Build history of the part. All positions in model axes, mm. A direction names the side the tool comes from. Give positions to 0.01 mm unless a question says otherwise; leave off trailing zeros. Write each loop counter-clockwise with the first axis right and the second up, starting at its lowest first coordinate (ties: lowest second). Pieces come first, ordered by that corner, then holes. Notation, with made-up numbers: (78, 89.5) -> (86, 89.5) arc R37 ccw to (86, 126.5) -> close; hole circle Ø8 at (17, 73). An arc over 180 degrees is marked (long way). One line per question, with ' | ' between items. Start each with the question number.
(1) Band-saw the part on B-B, the plane z = 0. Give the cut face in (x, y), and give its area (3 significant figures).
(2) Band-saw the part on C-C, the plane y = 5.5. Give the cut face in (x, z), and give its area (3 significant figures).
(3) Tool access for faces 4 (the cylindrical face through (0.03, 3.44, 7.66)), 5 (the flat face through (8, 14, -1.102)), 6 (the cylindrical face through (-5.323, 13.804, 2.769)): list every direction of +Z, -Z, +X, -X, +Y, -Y with a clear straight run to the whole face (end or side of a thin tool).
(4) Pull direction X, two halves, no side cores. Call faces 1 (the cylindrical face through (-0.027, 23.206, -7.713)), 2 (the cylindrical face through (-7.72, 3.79, -0.02)), 3 (the cylindrical face through (-3.639, 13.819, 8.776)): released by +X, released by -X, zero draft, split by the parting line, or undercut.
(5) Pin check, flat tips, straight feed: P1, Ø5, axis at x = 2.5, y = 7.5, coming from the -Z side; P2, Ø1.8, axis at x = -8.5, y = 15.5, coming from the -Z side; P3, Ø8, axis at y = 13, z = 5.5, coming from the -X side; P4, Ø2, axis at x = 4.5, z = 1, coming from the +Y side. Stop position of each tip, or through.
(6) Drill centre lines: probe 1 along X at (y, z) = (15.5, -7.5); probe 2 along Z at (x, y) = (-7.5, 11.25); probe 3 along Z at (x, y) = (2.25, 25.25). Where is each one in solid material? Low to high. Write a range as from..to.
(7) Band-saw the part on A-A, the plane x = 0. Give the cut face in (y, z), and give its area (3 significant figures).
from build123d import *

# Parameters (mm, degrees)
SKETCH_1_R               = 9.5
SKETCH_1_R_2             = 6
EXTRUDE_1_DEPTH          = 28
FILLET_1_R               = 1.1
CUT_EXTRUDE_1_DEPTH      = 15
CUT_EXTRUDE_1_DEPTH_BACK = 17
CUT_EXTRUDE_2_DEPTH      = 17
CUT_EXTRUDE_2_DEPTH_BACK = 17


with BuildPart() as part:
    # Эскиз1 → Бобышка-Вытянуть1 (new body)
    with BuildSketch(Plane(origin=(0, 0, 0), x_dir=(1, 0, 0), z_dir=(0, 1, 0))):
        with Locations(Location((0, 0, 0), (0, 0, 270))):
            Circle(SKETCH_1_R)
        with Locations(Location((0, 0, 0), (0, 0, 270))):
            Circle(SKETCH_1_R_2, mode=Mode.SUBTRACT)
    extrude(amount=EXTRUDE_1_DEPTH)

    # Скругление1
    fillet_1_edges = [part.edges().sort_by_distance(p)[0] for p in [
        (0, 0, -9.5),
        (0, 28, -9.5),
    ]]
    fillet(fillet_1_edges, radius=FILLET_1_R)

    # Эскиз2 → Вырез-Вытянуть1 (cut, two sides: drawn at the far end of the back side and taken through both)
    with BuildSketch(Plane.XY.offset(-CUT_EXTRUDE_1_DEPTH_BACK)):
        with BuildLine():
            Line((1.218447758, 21.987601969), (1.218447758, 4.658567189))
            ThreePointArc((1.218447758, 4.658567189), (0, 3.440119431), (-1.218447758, 4.658567189))
            Line((-1.218447758, 4.658567189), (-1.218447758, 21.987601969))
            ThreePointArc((-1.218447758, 21.987601969), (0, 23.206049726), (1.218447758, 21.987601969))
        make_face()
    extrude(amount=CUT_EXTRUDE_1_DEPTH + CUT_EXTRUDE_1_DEPTH_BACK, mode=Mode.SUBTRACT)

    # Эскиз3 → Вырез-Вытянуть2 (cut, two sides: drawn at the far end of the back side and taken through both)
    with BuildSketch(Plane(origin=(0, 0, 0), x_dir=(0, 0, -1), z_dir=(1, 0, 0)).offset(-CUT_EXTRUDE_2_DEPTH_BACK)):
        with BuildLine():
            Line((1.102405114, 22.761219593), (1.102405114, 4.890652477))
            ThreePointArc((1.102405114, 4.890652477), (0, 3.788247362), (-1.102405114, 4.890652477))
            Line((-1.102405114, 4.890652477), (-1.102405114, 22.761219593))
            ThreePointArc((-1.102405114, 22.761219593), (0, 23.863624707), (1.102405114, 22.761219593))
        make_face()
    extrude(amount=CUT_EXTRUDE_2_DEPTH + CUT_EXTRUDE_2_DEPTH_BACK, mode=Mode.SUBTRACT)


solid = part.part
Results:
1) outline: (-9.5, 1.1) arc R1.1 ccw to (-8.4, 0) -> (-6, 0) -> (-6, 3.79) -> (-9.5, 3.79) -> close; (-9.5, 23.86) -> (-6, 23.86) -> (-6, 28) -> (-8.4, 28) arc R1.1 ccw to (-9.5, 26.9) -> close; (6, 0) -> (8.4, 0) arc R1.1 ccw to (9.5, 1.1) -> (9.5, 3.79) -> (6, 3.79) -> close; (6, 23.86) -> (9.5, 23.86) -> (9.5, 26.9) arc R1.1 ccw to (8.4, 28) -> (6, 28) -> close | area: 54.4 mm²
2) outline: (-9.44, -1.1) arc R9.5 ccw to (-1.22, -9.42) -> (-1.22, -5.87) arc R6 cw to (-5.9, -1.1) -> close; (-9.44, 1.1) -> (-5.9, 1.1) arc R6 cw to (-1.22, 5.87) -> (-1.22, 9.42) arc R9.5 ccw to start; (1.22, -9.42) arc R9.5 ccw to (9.44, -1.1) -> (5.9, -1.1) arc R6 cw to (1.22, -5.87) -> close; (1.22, 5.87) arc R6 cw to (5.9, 1.1) -> (9.44, 1.1) arc R9.5 ccw to (1.22, 9.42) -> close | area: 138 mm²
3) face 4: +Z, -Z | face 5: +X, -X | face 6: +Y, -Y
4) face 1: undercut | face 2: zero draft | face 3: split by the parting line
5) P1: stops at z = -9.42 | P2: stops at z = -5.7 | P3: stops at x = -9.38 | P4: passes through
6) probe 1: x = -5.83..-1.22, 1.22..5.83 | probe 2: z = -5.83..-1.1, 1.1..5.83 | probe 3: z = -9.23..-5.56, 5.56..9.23
7) outline: (0, -8.4) arc R1.1 ccw to (1.1, -9.5) -> (3.44, -9.5) -> (3.44, -6) -> (0, -6) -> close; (0, 6) -> (3.44, 6) -> (3.44, 9.5) -> (1.1, 9.5) arc R1.1 ccw to (0, 8.4) -> close; (23.21, -9.5) -> (26.9, -9.5) arc R1.1 ccw to (28, -8.4) -> (28, -6) -> (23.21, -6) -> close; (23.21, 6) -> (28, 6) -> (28, 8.4) arc R1.1 ccw to (26.9, 9.5) -> (23.21, 9.5) -> close | area: 56.6 mm²
